```python
from build123d import *

# Parameters (mm, degrees)
CROQUIS1_R              = 11.115
CROQUIS1_R_2            = 3.175
SALIENTE_EXTRUIR1_DEPTH = 5


with BuildPart() as part:
    # Croquis1 → Saliente-Extruir1 (new body)
    with BuildSketch(Plane.XY):
        with BuildLine():
            Line((-31.855258333, 6.072933107), (-4.416099167, 14.455493528))
            ThreePointArc((-4.416099167, 14.455493528), (0, 15.115), (4.416099167, 14.455493528))
            Line((4.416099167, 14.455493528), (31.855258333, 6.072933107))
            ThreePointArc((31.855258333, 6.072933107), (36.35, 0), (31.855258333, -6.072933107))
            Line((31.855258333, -6.072933107), (4.416099167, -14.455493528))
            ThreePointArc((4.416099167, -14.455493528), (0, -15.115), (-4.416099167, -14.455493528))
            Line((-4.416099167, -14.455493528), (-31.855258333, -6.072933107))
            ThreePointArc((-31.855258333, -6.072933107), (-36.35, 0), (-31.855258333, 6.072933107))
        make_face()
        Circle(CROQUIS1_R, mode=Mode.SUBTRACT)
        with Locations((-30, 0)):
            Circle(CROQUIS1_R_2, mode=Mode.SUBTRACT)
        with Locations(Location((30, 0, 0), (0, 0, 180))):
            Circle(CROQUIS1_R_2, mode=Mode.SUBTRACT)
    extrude(amount=SALIENTE_EXTRUIR1_DEPTH)


solid = part.part
```
Input: part model. Units: mm. Frame: model coordinates. Give positions to 0.01 mm unless a question says otherwise; leave off trailing zeros. Order: outer loops, then holes, each group sorted by start corner. A loop starts at its lowest first (then second) coordinate and runs counter-clockwise, first axis right, second up. Notation, with made-up numbers: M -28.5,84.5 L 29.5,84.5 A12 cw 29.5,98.5 Z; hole C 58.25,-16 d3. An arc over 180 degrees is marked long. One line per question, with ' | ' between items.
1) Contact query for flat-ended pins moving along their axis: P1, Ø13.5, axis at x = 0, y = 0, coming from the +Z side; P2, Ø3, axis at y = -2.5, z = 1.5, coming from the +X side; P3, Ø1, axis at x = 13.5, z = 1, coming from the +Y side. Output: stop coordinate, or through.
Filled in:
P1: passes through | P2: stops at x = 36.27 | P3: stops at y = 11.83
2) Draft query along Y for faces 1 (the face through (-8, -10, 5)), 2 (the face through (0.063, -15.115, 2.465)), 3 (the face through (33.17, -0.14, 2.46)). Return one class per face: pulls with the +Y half, pulls with the -Y half, needs draft (parallel to the pull), parting line crosses it, or undercut.
Filled in:
face 1: needs draft | face 2: pulls with the -Y half | face 3: undercut
3) Section C-C on y = 0. Output: boundary loops of the cut face in (x, z) (3 decimals).
Filled in:
outline: M -36.35,0 L -33.175,0 L -33.175,5 L -36.35,5 Z; M -26.825,0 L -11.115,0 L -11.115,5 L -26.825,5 Z; M 11.115,0 L 26.825,0 L 26.825,5 L 11.115,5 Z; M 33.175,0 L 36.35,0 L 36.35,5 L 33.175,5 Z
4) Ray query, L1, parallel to Y at x = -0.5, z = 4.75; L2, parallel to X at y = -1, z = 3; L3, parallel to X at y = 4, z = 3.55. Return the intervals inside material, ascending.
Filled in:
L1: y = -15.11 to -11.1, 11.1 to 15.11 | L2: x = -36.27 to -33.01, -26.99 to -11.07, 11.07 to 26.99, 33.01 to 36.27 | L3: x = -34.93 to -10.37, 10.37 to 34.93
5) Section B-B on x = 0. Output: boundary loops of the cut face in (y, z) (3 decimals).
Filled in:
outline: M -15.115,0 L -11.115,0 L -11.115,5 L -15.115,5 Z; M 11.115,0 L 15.115,0 L 15.115,5 L 11.115,5 Z
6) Section D-D on y = 4.5. Output: boundary loops of the cut face in (x, z), and give its area (3 significant figures).
Filled in:
outline: M -34.48,0 L -10.16,0 L -10.16,5 L -34.48,5 Z; M 10.16,0 L 34.48,0 L 34.48,5 L 10.16,5 Z | area: 243 mm2
7) Section A-A on z = 3.55. State how many separate pieces and enclosed holes the cut face has, and give its area (3 significant figures).
Filled in:
separate pieces: 1 | enclosed holes: 3 | area: 1,020 mm2
